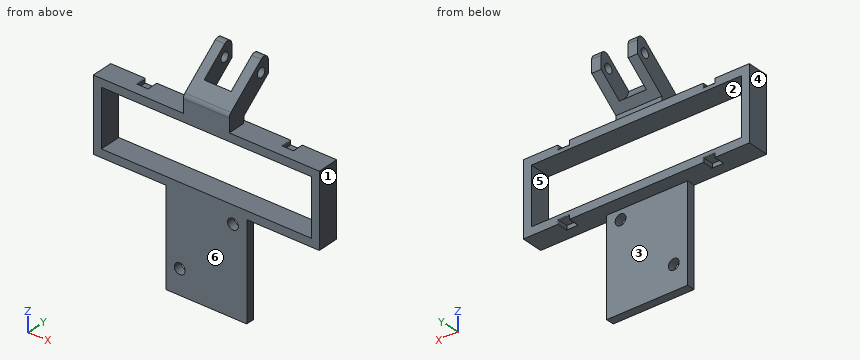
from build123d import *

# Parameters (mm, degrees)
SKETCH5_W           = 77.7
SKETCH5_H           = 21.028
BOSS_EXTRUDE3_DEPTH = 8
SKETCH6_W           = 30
SKETCH6_H           = 35.57641867
CUT_EXTRUDE4_DEPTH  = 5
SKETCH10_R          = 1.7
CUT_EXTRUDE5_DEPTH  = 17
FILLET4_R           = 2
FILLET5_R           = 2
CHAMFER1_START      = 6.5
CHAMFER1_DEPTH      = 17
SKETCH11_R          = 10
CUT_EXTRUDE6_DEPTH  = 5
SKETCH12_R          = 2
CUT_EXTRUDE7_DEPTH  = 3
SKETCH13_W          = 4
SKETCH13_H          = 1.5
CUT_EXTRUDE8_DEPTH  = 4
FILLET6_R           = 0.25


with BuildPart() as part:
    # Sketch5 → Boss-Extrude3 (new body)
    with BuildSketch(Plane(origin=(0, 0, 0), x_dir=(1, 0, 0), z_dir=(0, 1, 0))):
        Polygon((30, -35.57641867), (56.85, -35.57641867), (56.85, -62.60441867), (-26.85, -62.60441867), (-26.85, -35.57641867), (0, -35.57641867), (0, 0), (30, 0), align=None)
        with Locations((15, -49.09041867)):
            Rectangle(SKETCH5_W, SKETCH5_H, mode=Mode.SUBTRACT)
    extrude(amount=BOSS_EXTRUDE3_DEPTH)

    # Sketch6 → Cut-Extrude4 (cut)
    with BuildSketch(Plane(origin=(0, 8, 0), x_dir=(1, 0, 0), z_dir=(0, 1, 0))):
        with Locations((15, -17.788209335)):
            Rectangle(SKETCH6_W, SKETCH6_H)
    extrude(amount=-CUT_EXTRUDE4_DEPTH, mode=Mode.SUBTRACT)

    # Sketch7 → Loft1 section 0
    with BuildSketch(Plane.XZ):
        with BuildLine():
            Line((6.5, 59.60441867), (23.5, 59.60441867))
            Line((23.5, 59.60441867), (23.5, 68.60441867))
            Line((23.5, 68.60441867), (6.5, 68.60441867))
            Line((6.5, 68.60441867), (6.5, 59.60441867))
        make_face()
    # Sketch9 → Loft1 section 1
    with BuildSketch(Plane(origin=(0, 18, 0), x_dir=(-1, 0, 0), z_dir=(0, -1, 0))):
        with BuildLine():
            Line((-23.5, -83.10441867), (-6.5, -83.10441867))
            Line((-6.5, -83.10441867), (-6.5, -74.10441867))
            Line((-6.5, -74.10441867), (-23.5, -74.10441867))
            Line((-23.5, -74.10441867), (-23.5, -83.10441867))
        make_face()
    loft()

    # Sketch10 → Cut-Extrude5 (cut)
    with BuildSketch(Plane(origin=(23.5, 0, 0), x_dir=(0, 0, -1), z_dir=(1, 0, 0))):
        with Locations(Location((-75.953844744, 14.709632368, 0), (0, 0, 90))):
            Circle(SKETCH10_R)
    extrude(amount=-CUT_EXTRUDE5_DEPTH, mode=Mode.SUBTRACT)

    # Fillet4
    fillet4_edges = [part.edges().sort_by_distance(p)[0] for p in [
        (15, 0, 68.60441867),
    ]]
    fillet(fillet4_edges, radius=FILLET4_R)

    # Fillet5
    fillet5_edges = [part.edges().sort_by_distance(p)[0] for p in [
        (15, 18, 83.10441867),
    ]]
    fillet(fillet5_edges, radius=FILLET5_R)

    # Chamfer1: read off the stored shape, not the designer's step
    # Chamfer1 outline → Chamfer1 (add)
    with BuildSketch(Plane.YZ.offset(CHAMFER1_START)):
        Polygon((6.568919305, 62.60441867), (6.839153567, 65.113736821), (3.724137931, 62.60441867), align=None)
    extrude(amount=CHAMFER1_DEPTH)

    # Sketch11 → Cut-Extrude6 (cut, symmetric)
    with BuildSketch(Plane(origin=(15, 0, 0), x_dir=(0, 0, -1), z_dir=(1, 0, 0))):
        with Locations((-75.953844744, 14.709632368)):
            Circle(SKETCH11_R)
    extrude(amount=CUT_EXTRUDE6_DEPTH, both=True, mode=Mode.SUBTRACT)

    # Sketch12 → Cut-Extrude7 (cut)
    with BuildSketch(Plane(origin=(0, 3, 0), x_dir=(1, 0, 0), z_dir=(0, 1, 0))):
        with Locations(Location((24.85, -32.02641867, 0), (0, 0, 270))):
            Circle(SKETCH12_R)
        with Locations(Location((5.15, -9.12641867, 0), (0, 0, 270))):
            Circle(SKETCH12_R)
    extrude(amount=-CUT_EXTRUDE7_DEPTH, mode=Mode.SUBTRACT)

    # Sketch13 → Cut-Extrude8 (cut)
    with BuildSketch(Plane(origin=(0, 8, 0), x_dir=(1, 0, 0), z_dir=(0, 1, 0))):
        with Locations((-11.925, -36.32641867)):
            Rectangle(SKETCH13_W, SKETCH13_H)
        with Locations((-11.925, -61.85441867)):
            Rectangle(SKETCH13_W, SKETCH13_H)
        with Locations((41.925, -61.85441867)):
            Rectangle(SKETCH13_W, SKETCH13_H)
        with Locations((41.925, -36.32641867)):
            Rectangle(SKETCH13_W, SKETCH13_H)
    extrude(amount=-CUT_EXTRUDE8_DEPTH, mode=Mode.SUBTRACT)

    # Fillet6
    fillet6_edges = [part.edges().sort_by_distance(p)[0] for p in [
        (-9.925, 6, 62.60441867),
        (-13.925, 6, 62.60441867),
        (-9.925, 8, 61.85441867),
        (-11.925, 8, 61.10441867),
        (-13.925, 8, 61.85441867),
        (39.925, 6, 35.57641867),
        (43.925, 6, 35.57641867),
        (39.925, 8, 36.32641867),
        (41.925, 8, 37.07641867),
        (43.925, 8, 36.32641867),
        (39.925, 6, 62.60441867),
        (43.925, 6, 62.60441867),
        (39.925, 8, 61.85441867),
        (43.925, 8, 61.85441867),
        (41.925, 8, 61.10441867),
        (-9.925, 6, 35.57641867),
        (-13.925, 6, 35.57641867),
        (-9.925, 8, 36.32641867),
        (-13.925, 8, 36.32641867),
        (-11.925, 8, 37.07641867),
    ]]
    fillet(fillet6_edges, radius=FILLET6_R)


solid = part.part
Model file for the job. Use its own axes, mm. Face numbers are marked on the shaded views. A direction names the side the tool comes from. Give positions to 0.01 mm unless a question says otherwise; leave off trailing zeros. Order: outer loops, then holes, each group sorted by start corner. A loop starts at its lowest first (then second) coordinate and runs counter-clockwise, first axis right, second up. Notation, with made-up numbers: (74.25, -3.75) - (114.25, -3.75) arc R21 cw to (114.25, 1.25) - close; hole circle Ø1 at (55.25, -10.5). An arc over 180 degrees is marked (long way). Write item = value, one per line. Start each with the question number.
1. Drop flat-ended pins along their axis: P1, Ø5, axis at x = 37, z = 41.5, coming from the -Y side; P2, Ø4, axis at x = -12, y = 5.5, coming from the -Z side; P3, Ø2.5, axis at x = 2.5, y = 5, coming from the +Z side; P4, Ø9, axis at y = 5, z = 75, coming from the +X side. Give the stop position or say it passes through.
2. Probe line 1 along Z through (x, y) = (46.5, 6.5); line 2 along Y through (x, z) = (1.5, 10); line 3 along Z through (x, y) = (8, 15). List the from-to ranges inside material, lowest first.
3. Which spindle directions (+Z, -Z, +X, -X, +Y, -Y) get a long thin tool onto all of the face, cutting with end or side? Do the marked faces 1, 2 and 3. Say none if no direction does.
4. Cut at B-B, the plane x = 5.15. List the corners of the cut face in (y, z), and give its area (3 significant figures).
5. Cut at C-C, the plane z = 56. List the corners of the cut face in (x, y).
6. Cut at A-A, the plane x = -17.5. List the corners of the cut face in (y, z).
7. Two-plate mould, pull along X, no slides. Class the marked faces 4, 5 and 6: pulls with the +X half, pulls with the -X half, needs draft (parallel to the pull), parting line crosses it, or undercut.
Taken from the geometry:
q1.P1 = through
q1.P2 = 35.58
q1.P3 = 62.6
q1.P4 = 23.5
q2.line_1 = 35.58 to 38.58, 59.6 to 62.6
q2.line_2 = 0 to 3
q2.line_3 = 71.69 to 74.28, 77.63 to 80.66
q3.face_1 = +Z, -Z, +X, +Y, -Y
q3.face_2 = +Y, -Y
q3.face_3 = -Z, +X, -X, +Y
q4.outline = (0, 0) - (3, 0) - (3, 7.13) - (0, 7.13) - close; (0, 11.13) - (3, 11.13) - (3, 35.58) - (8, 35.58) - (8, 38.58) - (0, 38.58) - close; (0, 59.6) - (8, 59.6) - (8, 62.6) - (0, 62.6) - close
q4.area = 143 mm²
q5.outline = (-26.85, 0) - (-23.85, 0) - (-23.85, 8) - (-26.85, 8) - close; (53.85, 0) - (56.85, 0) - (56.85, 8) - (53.85, 8) - close
q6.outline = (0, 35.58) - (8, 35.58) - (8, 38.58) - (0, 38.58) - close; (0, 59.6) - (8, 59.6) - (8, 62.6) - (0, 62.6) - close
q7.face_4 = pulls with the -X half
q7.face_5 = undercut
q7.face_6 = needs draft
